from build123d import *

# Parameters (mm, degrees)
BOSS_EXTRUDE1_DEPTH = 22.5
SKETCH3_R           = 4
CUT_EXTRUDE1_DEPTH  = 51.204979833
SKETCH3_4_R         = 6.5
SKETCH3_4_R_2       = 4
CUT_EXTRUDE2_DEPTH  = 6
FILLET1_R           = 10
FILLET2_R           = 5
FILLET4_R           = 2
CHAMFER1_SIZE       = 1


# Some blends are built 0.0001 mm under size
with BuildPart() as part:
    # Sketch1 → Boss-Extrude1 (new, symmetric)
    with BuildSketch(Plane.XY):
        Polygon((-22.7, -12.5), (2.7, -12.5), (2.7, 5.5), (42.3, 5.5), (42.3, 12.5), (-2.7, 12.5), (-2.7, -2.5), (-22.7, -2.5), align=None)
    extrude(amount=BOSS_EXTRUDE1_DEPTH, both=True)

    # Sketch3 → Cut-Extrude1 (cut, through all)
    with BuildSketch(Plane(origin=(0, -2.5, 0), x_dir=(1, 0, 0), z_dir=(0, 1, 0))):
        with Locations(Location((-10, -12.7, 0), (0, 0, 180))):
            Circle(SKETCH3_R)
    cut_extrude1 = extrude(amount=-CUT_EXTRUDE1_DEPTH, mode=Mode.SUBTRACT)

    # Sketch3<4> → Cut-Extrude2 (cut)
    with BuildSketch(Plane(origin=(0, -2.5, 0), x_dir=(1, 0, 0), z_dir=(0, 1, 0))):
        with Locations(Location((-10, -12.7, 0), (0, 0, 180))):
            Circle(SKETCH3_4_R)
        with Locations(Location((-10, -12.7, 0), (0, 0, 180))):
            Circle(SKETCH3_4_R_2, mode=Mode.SUBTRACT)
    cut_extrude2 = extrude(amount=-CUT_EXTRUDE2_DEPTH, mode=Mode.SUBTRACT)

    # Mirror1: Cut-Extrude1, Cut-Extrude2 across plane
    add(cut_extrude1.mirror(Plane.XY), mode=Mode.SUBTRACT)
    add(cut_extrude2.mirror(Plane.XY), mode=Mode.SUBTRACT)

    # Fillet1
    # the kernel refuses this fillet: 10 mm, written as the material it adds along each edge
    with BuildSketch(Plane(origin=(-2.7, -2.5, 22.5), x_dir=(0, 1, 0), z_dir=(0, 0, -1))) as fillet1_piece_1_section:
        with BuildLine():
            CenterArc((FILLET1_R, -FILLET1_R), FILLET1_R, 90, 90)
            Line((0, -FILLET1_R), (0, 0))
            Line((0, 0), (FILLET1_R, 0))
        make_face()
    fillet1_piece_1 = extrude(amount=45, mode=Mode.PRIVATE)
    fillet1_piece_1 = fillet1_piece_1 - Plane(origin=(-10, 0.155378063, -12.7), x_dir=(-1, 0, 0), z_dir=(0, 1, 0)) * Cylinder(6.5, 130, mode=Mode.PRIVATE)
    fillet1_piece_1 = fillet1_piece_1 - Plane(origin=(-10, 0.155378063, 12.7), x_dir=(-1, 0, 0), z_dir=(0, 1, 0)) * Cylinder(6.5, 130, mode=Mode.PRIVATE)
    add(fillet1_piece_1)

    # Fillet2
    fillet2_edges = [part.edges().sort_by_distance(p)[0] for p in [
        (2.7, 5.5, 0),
        (-22.7, -2.5, 0),
        (-2.7, 12.5, 0),
    ]]
    fillet(fillet2_edges, radius=FILLET2_R - 0.0001)  # a hair under: the kernel refuses the full size

    # Fillet4
    fillet4_edges = [part.edges().sort_by_distance(p)[0] for p in [
        (42.3, 12.5, 0),
        (42.3, 5.5, 0),
    ]]
    fillet(fillet4_edges, radius=FILLET4_R)

    # Chamfer1
    chamfer1_edges = [part.edges().sort_by_distance(p)[0] for p in [
        (2.7, -5.99995, -22.5),
        (-10, -12.5, -22.5),
        (2.7, -5.99995, 22.5),
        (-15.20005, -2.5, -22.5),
        (-15.20005, -2.5, 22.5),
        (-5.628932188, 0.428932188, -22.5),
        (-5.628932188, 0.428932188, 22.5),
        (-22.7, -9.99995, -22.5),
        (-22.7, -9.99995, 22.5),
        (23.99995, 5.5, -22.5),
        (-1.235563195, 11.035563195, -22.5),
        (-21.235563195, -3.964436805, -22.5),
        (23.99995, 5.5, 22.5),
        (-1.235563195, 11.035563195, 22.5),
        (-21.235563195, -3.964436805, 22.5),
        (4.164436805, 4.035563195, -22.5),
        (4.164436805, 4.035563195, 22.5),
        (21.29995, 12.5, -22.5),
        (21.29995, 12.5, 22.5),
        (42.3, 9, -22.5),
        (41.714213562, 6.085786438, -22.5),
        (41.714213562, 11.914213562, -22.5),
        (42.3, 9, 22.5),
        (41.714213562, 6.085786438, 22.5),
        (41.714213562, 11.914213562, 22.5),
        (-10, -12.5, 22.5),
    ]]
    chamfer(chamfer1_edges, length=CHAMFER1_SIZE)


solid = part.part
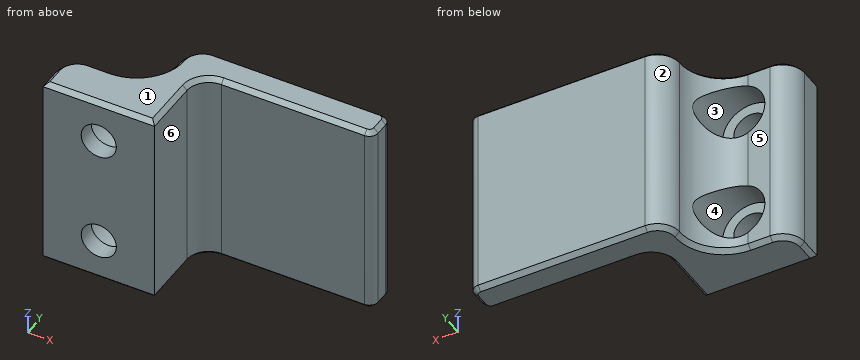
The model under review builds one solid part; all positions refer to its coordinate system, in mm. Face numbers are marked on the shaded views. A direction names the side the tool comes from. Round coordinates to 2 decimals unless told otherwise and drop trailing zeros. Write each loop counter-clockwise with the first axis right and the second up, starting at its lowest first coordinate (ties: lowest second). Pieces come first, ordered by that corner, then holes. Notation, with made-up numbers: (46.5, -11.75) - (86.5, -11.75) arc R22 ccw to (86.5, 21.25) - close; hole circle Ø6 at (67, -25). An arc over 180 degrees is marked (long way). One line per item, written item: value. Start each with the question number.
1. Consider section D-D on x = -10.5. State how many separate pieces and enclosed holes the cut face has, and give its area (3 significant figures).
2. Consider section B-B on x = 28.5. Write out the cut boundary in (y, z).
3. Machinability: for the marked faces 4, 5 and 6, which of the approach directions +Z, -Z, +X, -X, +Y, -Y give a long, thin tool a straight path to every point of the face, cutting with its end or side? Answer none if there is none.
4. Clearance check with flat-ended pins moving along their axes: P1, Ø8, axis at x = 26.5, z = 1, coming from the -Y side; P2, Ø7, axis at x = -10, z = 12.7, coming from the +Y side; P3, Ø14.5, axis at y = -7.5, z = 2.5, coming from the +X side; P4, Ø2.5, axis at x = -16, z = 1, coming from the +Y side. State where each tip first meets the part, or that it passes through.
5. To check wall thickness, follow L1, parallel to Z at x = -10, y = -5; L2, parallel to Z at x = -10, y = -10.65; L3, parallel to X at y = -10.85, z = -12.7. State the ranges of each line that lie inside material, in increasing order. Write a range as from..to.
6. The part is to be moulded in two halves that separate along Z. For the marked faces 1, 2 and 3, say which applies: released by +Z, released by -Z, zero draft, split by the parting line, or undercut.
Checks:
1. separate pieces: 3
1. enclosed holes: 0
1. area: 234 mm^2
2. outline: (5.5, -21.5) - (6.5, -22.5) - (11.5, -22.5) - (12.5, -21.5) - (12.5, 21.5) - (11.5, 22.5) - (6.5, 22.5) - (5.5, 21.5) - close
3. face 4: +Y
3. face 5: +Z, -Z, -X, +Y
3. face 6: +Z, -Z, +X, -Y
4. P1: stops at y = 5.5
4. P2: passes through
4. P3: stops at x = 2.7
4. P4: stops at y = -2.5
5. L1: z = -22.5..-19.2, -6.2..6.2, 19.2..22.5
5. L2: z = -22.5..-16.7, -8.7..8.7, 16.7..22.5
5. L3: x = -22.7..-14, -6..2.7
6. face 1: released by +Z
6. face 2: zero draft
6. face 3: undercut
